Source: three-view drawing plus pictorial views. Frame: mm from the lowest corner of the part. Coordinates: 2 decimals unless noted, no trailing zeros. Order: outer loops, then holes, each group sorted by start corner. A loop starts at its lowest first (then second) coordinate and runs counter-clockwise, first axis right, second up. Notation, with made-up numbers: (63.5, 14.5) - (68.5, 14.5) arc R30 cw to (68.5, 38.5) - close; hole circle Ø11 at (81, 4.5). An arc over 180 degrees is marked (long way). One line per question, with ' | ' between items.
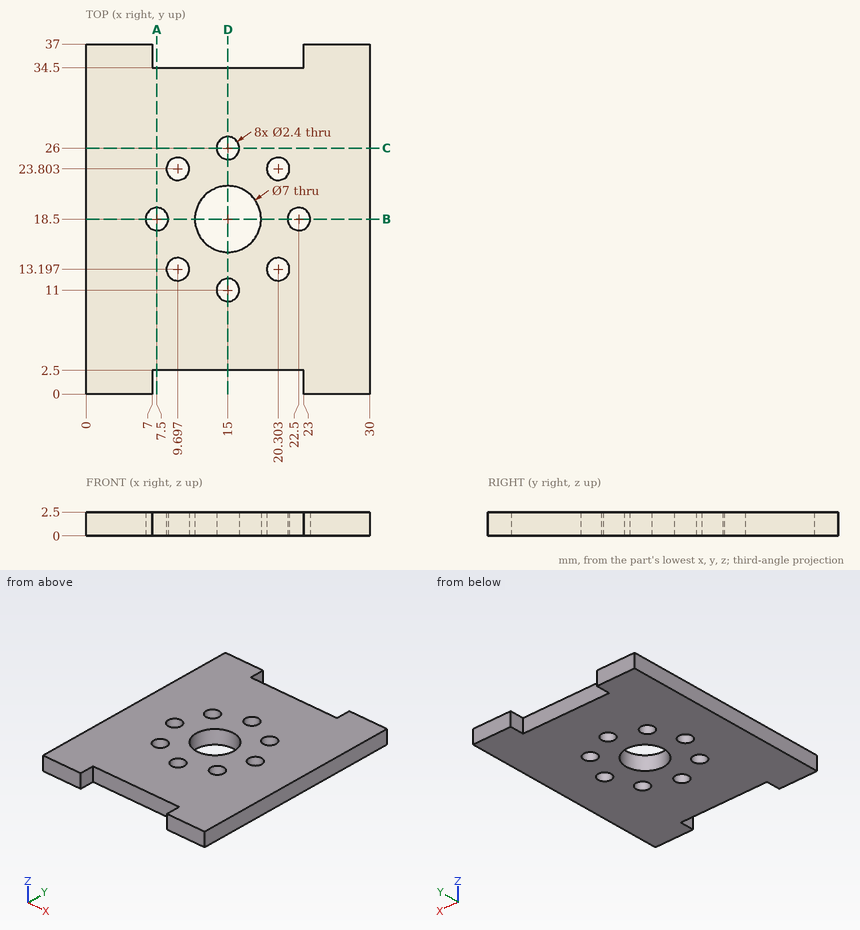
(1) Material intervals for L1, parallel to Y at x = 15, z = 1.4; L2, parallel to X at y = 13, z = 0.7; L3, parallel to Y at x = 15.75, z = 0.4, sorted ascending. Write a range as from..to.
Taken from the geometry:
L1: y = 2.5..9.8, 12.2..15, 22..24.8, 27.2..34.5 | L2: x = 0..8.51, 10.88..19.12, 21.49..30 | L3: y = 2.5..10.06, 11.94..15.08, 21.92..25.06, 26.94..34.5
(2) Cut plane A-A (x = 7.5). Return the cut outline in (y, z).
Taken from the geometry:
outline: (2.5, 0) - (17.3, 0) - (17.3, 2.5) - (2.5, 2.5) - close; (19.7, 0) - (34.5, 0) - (34.5, 2.5) - (19.7, 2.5) - close
(3) Pin query (flat end, axial travel): P1, Ø1.2, axis at x = 12, z = 1, coming from the -Y side; P2, Ø2, axis at x = 15, y = 11, coming from the -Z side; P3, Ø1.5, axis at x = 15, z = 2, coming from the +Y side. Return the tip coordinate at first contact, or that it passes through.
Taken from the geometry:
P1: stops at y = 2.5 | P2: passes through | P3: stops at y = 34.5
(4) Cut plane C-C (y = 26). Return the cut outline in (x, z).
Taken from the geometry:
outline: (0, 0) - (13.8, 0) - (13.8, 2.5) - (0, 2.5) - close; (16.2, 0) - (30, 0) - (30, 2.5) - (16.2, 2.5) - close
(5) Cut plane D-D (x = 15). Return the cut outline in (y, z), and give its area (3 significant figures).
Taken from the geometry:
outline: (2.5, 0) - (9.8, 0) - (9.8, 2.5) - (2.5, 2.5) - close; (12.2, 0) - (15, 0) - (15, 2.5) - (12.2, 2.5) - close; (22, 0) - (24.8, 0) - (24.8, 2.5) - (22, 2.5) - close; (27.2, 0) - (34.5, 0) - (34.5, 2.5) - (27.2, 2.5) - close | area: 50.5 mm²
(6) Cut plane B-B (y = 18.5). Return the cut outline in (x, z), and give its area (3 significant figures).
Taken from the geometry:
outline: (0, 0) - (6.3, 0) - (6.3, 2.5) - (0, 2.5) - close; (8.7, 0) - (11.5, 0) - (11.5, 2.5) - (8.7, 2.5) - close; (18.5, 0) - (21.3, 0) - (21.3, 2.5) - (18.5, 2.5) - close; (23.7, 0) - (30, 0) - (30, 2.5) - (23.7, 2.5) - close | area: 45.5 mm²
